```python
from build123d import *

# Parameters (mm, degrees)
F0_W     = 76.2
F0_H     = 152.4
F1_DEPTH = 25.4
F2_W     = 20.32
F2_H     = 20.32
F3_DEPTH = 12.7


with BuildPart() as f1:
    # F0 (on Top) → F1 (new body)
    with BuildSketch(Plane.XY):
        Rectangle(F0_W, F0_H)
    extrude(amount=-F1_DEPTH)

    # F2 (on face) → F3 (cut)
    with BuildSketch(Plane.XY):
        with Locations((-18.621309, 61.657559)):
            Rectangle(F2_W, F2_H)
        with Locations((18.621309, 61.657559)):
            Rectangle(F2_W, F2_H)
        with Locations((18.621309, -61.657559)):
            Rectangle(F2_W, F2_H)
        with Locations((-18.621309, -61.657559)):
            Rectangle(F2_W, F2_H)
        with Locations((-18.840398, 19.318015)):
            Rectangle(F2_W, F2_H)
        with Locations((18.840398, 19.318015)):
            Rectangle(F2_W, F2_H)
        with Locations((-18.840398, -19.318015)):
            Rectangle(F2_W, F2_H)
        with Locations((18.840398, -19.318015)):
            Rectangle(F2_W, F2_H)
    extrude(amount=-F3_DEPTH, mode=Mode.SUBTRACT)


solid = f1.part
```
Part model, mm, in its own coordinate system. A direction names the side the tool comes from. Round coordinates to 2 decimals unless told otherwise and drop trailing zeros. Write each loop counter-clockwise with the first axis right and the second up, starting at its lowest first coordinate (ties: lowest second). Pieces come first, ordered by that corner, then holes. Notation, with made-up numbers: M 75,88 L 84,88 A19 cw 84,108 Z; hole C -39.5,64 d8. An arc over 180 degrees is marked long. One line per question, with ' | ' between items.
(1) Pin check, flat tip, straight feed: pin 1 (6 mm diameter, centred on x = 15.5, y = 22.5, fed in from +Z). Stop position of the tip, or through.
Answer key:
pin 1: stops at z = -12.7
(2) Two-plate mould, pull along Y, no slides. Class faces 3 (the face through (-19, 29.478, -6)), 4 (the face through (-1, 1, 0)), 5 (the face through (-1, -76.2, -13)): released by +Y, released by -Y, zero draft, split by the parting line, or undercut.
Answer key:
face 3: undercut | face 4: zero draft | face 5: released by -Y
(3) Saw through at A-A on x = -21. Write the cut outline in (y, z).
Answer key:
outline: M -76.2,-25.4 L 76.2,-25.4 L 76.2,0 L 71.82,0 L 71.82,-12.7 L 51.5,-12.7 L 51.5,0 L 29.48,0 L 29.48,-12.7 L 9.16,-12.7 L 9.16,0 L -9.16,0 L -9.16,-12.7 L -29.48,-12.7 L -29.48,0 L -51.5,0 L -51.5,-12.7 L -71.82,-12.7 L -71.82,0 L -76.2,0 Z
(4) Saw through at C-C on z = -4.25. Count the separate pieces of the cut face and the enclosed holes in it, then the cut area to 3 significant figures.
Answer key:
separate pieces: 1 | enclosed holes: 8 | area: 8,310 mm^2
(5) Saw through at B-B on y = -18. Write the cut outline in (x, z), then the cut area to 3 significant figures.
Answer key:
outline: M -38.1,-25.4 L 38.1,-25.4 L 38.1,0 L 29,0 L 29,-12.7 L 8.68,-12.7 L 8.68,0 L -8.68,0 L -8.68,-12.7 L -29,-12.7 L -29,0 L -38.1,0 Z | area: 1,420 mm^2
(6) 3-axis set-ups, long thin cutter, end or side, ignore diameter. For faces 1 (the face through (-1, 76.2, -13)), 2 (the face through (-19, -19, -12.7)): which of +Z, -Z, +X, -X, +Y, -Y reach the whole face in a straight line?
Answer key:
face 1: +Z, -Z, +X, -X, +Y | face 2: +Z
(7) Probe line 1 along X through (y, z) = (-11.5, -2.25); line 2 along X through (y, z) = (-52.5, -7); line 3 along Z through (x, y) = (-22, 60). List the from-to ranges inside material, lowest first.
Answer key:
line 1: x = -38.1 to -29, -8.68 to 8.68, 29 to 38.1 | line 2: x = -38.1 to -28.78, -8.46 to 8.46, 28.78 to 38.1 | line 3: z = -25.4 to -12.7
